Check sheet for the drawn part. Datum: minimum x, y, z corner. Units: mm. A direction names the side the tool comes from. Give positions to 0.01 mm unless a question says otherwise; leave off trailing zeros. Order: outer loops, then holes, each group sorted by start corner. A loop starts at its lowest first (then second) coordinate and runs counter-clockwise, first axis right, second up. Notation, with made-up numbers: M 88,-15 L 129,-15 A7 cw 129,-6 Z; hole C -27.75,-35.75 d7. An arc over 180 degrees is marked long. Answer in a Markdown table with one row per item. Add a question column.
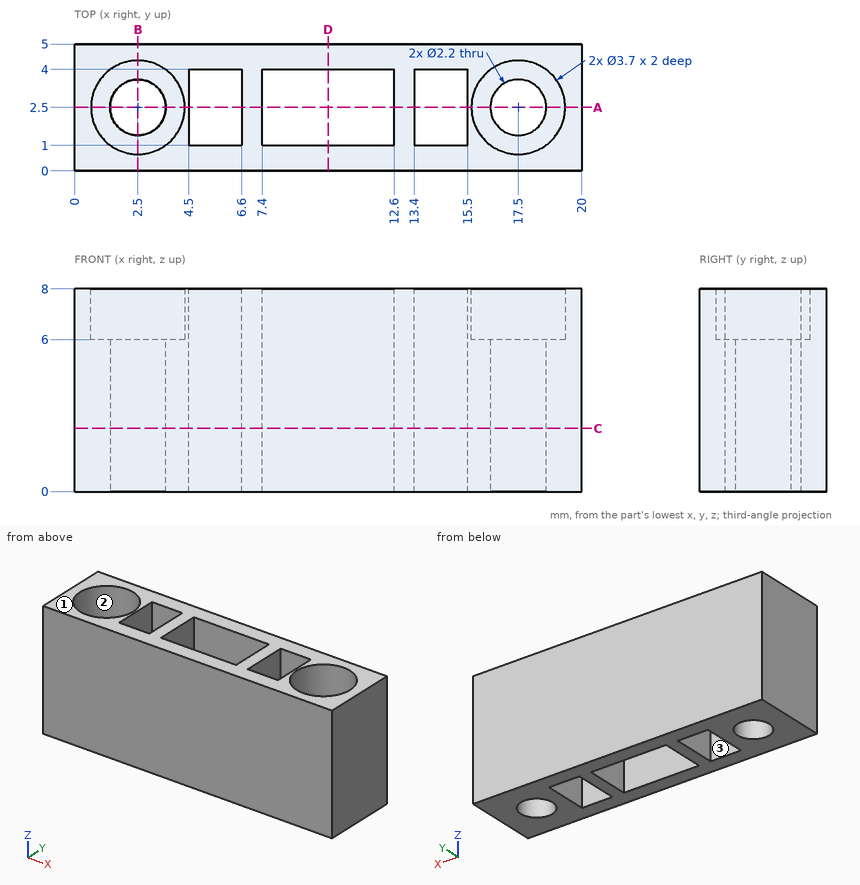
Q1. Tool access check on the marked faces 1, 2 and 3. Record the directions out of +Z, -Z, +X, -X, +Y, -Y that give a thin tool (end or side, any length) a straight path to the whole face; none if there is none.
Q2. Thickness scan on probe 1 along Y at (x, z) = (2.5, 7); probe 2 along X at (y, z) = (3.3, 2.25); probe 3 along Y at (x, z) = (17.5, 4.45). Record the ranges inside material, lowest first.
Q3. Cross-section at A-A (y = 2.5). State how many separate pieces and enclosed holes the cut face has, and give its area (3 significant figures).
Q4. Cross-section at C-C (z = 2.5). Record the boundary of the cut face in (x, y).
Q5. Cross-section at B-B (x = 2.5). Record the boundary of the cut face in (y, z), and give its area (3 significant figures).
Q6. Go/stop test with a flat-tipped pin: pin 1 (1.1 mm diameter, centred on x = 18, y = 3, fed in from +Z). Record where the tip stops, or that it passes through.
Q7. Cross-section at D-D (x = 10). Record the boundary of the cut face in (y, z).
Values follow:
| question | item | result |
|---|---|---|
| 1 | face 1 | +Z, +X, -X, +Y, -Y |
| 1 | face 2 | +Z |
| 1 | face 3 | +Z, -Z |
| 2 | probe 1 | 0 to 0.65, 4.35 to 5 |
| 2 | probe 2 | 0 to 1.75, 3.25 to 4.5, 6.6 to 7.4, 12.6 to 13.4, 15.5 to 16.75, 18.25 to 20 |
| 2 | probe 3 | 0 to 1.4, 3.6 to 5 |
| 3 | separate pieces | 6 |
| 3 | enclosed holes | 0 |
| 3 | area | 43.6 mm² |
| 4 | outline | M 0,0 L 20,0 L 20,5 L 0,5 Z; hole C 2.5,2.5 d2.2; hole M 4.5,1 L 6.6,1 L 6.6,4 L 4.5,4 Z; hole M 7.4,1 L 12.6,1 L 12.6,4 L 7.4,4 Z; hole M 13.4,1 L 15.5,1 L 15.5,4 L 13.4,4 Z; hole C 17.5,2.5 d2.2 |
| 5 | outline | M 0,0 L 1.4,0 L 1.4,6 L 0.65,6 L 0.65,8 L 0,8 Z; M 3.6,0 L 5,0 L 5,8 L 4.35,8 L 4.35,6 L 3.6,6 Z |
| 5 | area | 19.4 mm² |
| 6 | pin 1 | z = 6 |
| 7 | outline | M 0,0 L 1,0 L 1,8 L 0,8 Z; M 4,0 L 5,0 L 5,8 L 4,8 Z |
